Geometry: final body of the model. Coordinates: model frame, mm. Face numbers are marked on the shaded views. Round coordinates to 2 decimals unless told otherwise and drop trailing zeros. Loops run counter-clockwise (first coordinate to the right, second up) from the corner with the lowest first, then second, coordinate; pieces in that order, holes last. Notation, with made-up numbers: M -36,9 L 18,9 A13 ccw 18,17 Z; hole C 61,-14.75 d1. An arc over 180 degrees is marked long. Answer as a JSON object with one key per item and string values.
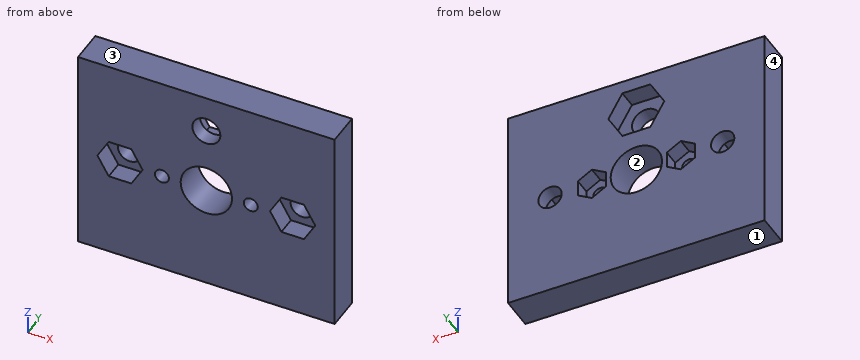
```python
from build123d import *

# Parameters (mm, degrees)
SKETCH1_W               = 55
SKETCH1_H               = 45
BOSS_EXTRUDE1_DEPTH     = 7.2
CUT_EXTRUDE1_DEPTH      = 37.253827384
CUT_EXTRUDE1_DEPTH_BACK = 37.253827384
SKETCH2_R               = 5.5
SKETCH2_R_2             = 2.5
SKETCH2_R_3             = 1.5
CUT_EXTRUDE2_DEPTH      = 3.5
CUT_EXTRUDE3_DEPTH      = 4
CUT_EXTRUDE4_DEPTH      = 37.253827384
CUT_EXTRUDE4_DEPTH_BACK = 37.253827384
SKETCH7_R               = 3
CUT_EXTRUDE5_DEPTH      = 4


with BuildPart() as part:
    # Sketch1 → Boss-Extrude1 (new body)
    with BuildSketch(Plane(origin=(0, 0, 0), x_dir=(1, 0, 0), z_dir=(0, 1, 0))):
        Rectangle(SKETCH1_W, SKETCH1_H)
    extrude(amount=BOSS_EXTRUDE1_DEPTH)

    # Sketch2 → Cut-Extrude1 (cut, two sides: drawn at the far end of the back side and taken through both)
    with BuildSketch(Plane(origin=(0, 7.2, 0), x_dir=(1, 0, 0), z_dir=(0, 1, 0)).offset(-CUT_EXTRUDE1_DEPTH_BACK)):
        with Locations(Location((0, 0, 0), (0, 0, 270))):
            Circle(SKETCH2_R)
        with Locations(Location((-18.5, 0, 0), (0, 0, 270))):
            Circle(SKETCH2_R_2)
        with Locations(Location((18.5, 0, 0), (0, 0, 270))):
            Circle(SKETCH2_R_2)
        with Locations(Location((-9.525, 0, 0), (0, 0, 270))):
            Circle(SKETCH2_R_3)
        with Locations(Location((9.525, 0, 0), (0, 0, 270))):
            Circle(SKETCH2_R_3)
    extrude(amount=CUT_EXTRUDE1_DEPTH + CUT_EXTRUDE1_DEPTH_BACK, mode=Mode.SUBTRACT)

    # Sketch3 → Cut-Extrude2 (cut)
    with BuildSketch(Plane(origin=(0, 7.2, 0), x_dir=(1, 0, 0), z_dir=(0, 1, 0))):
        Polygon((-9.525, 3.464101615), (-12.525, 1.732050808), (-12.525, -1.732050808), (-9.525, -3.464101615), (-6.525, -1.732050808), (-6.525, 1.732050808), align=None)
        Polygon((9.525, 3.464101615), (6.525, 1.732050808), (6.525, -1.732050808), (9.525, -3.464101615), (12.525, -1.732050808), (12.525, 1.732050808), align=None)
    extrude(amount=-CUT_EXTRUDE2_DEPTH, mode=Mode.SUBTRACT)

    # Sketch5 → Cut-Extrude3 (cut)
    with BuildSketch(Plane.XZ):
        Polygon((23.349742261, 0), (20.924871131, 4.2), (16.075128869, 4.2), (13.650257739, 0), (16.075128869, -4.2), (20.924871131, -4.2), align=None)
        Polygon((-13.650257739, 0), (-16.075128869, 4.2), (-20.924871131, 4.2), (-23.349742261, 0), (-20.924871131, -4.2), (-16.075128869, -4.2), align=None)
    extrude(amount=-CUT_EXTRUDE3_DEPTH, mode=Mode.SUBTRACT)

    # Sketch7 → Cut-Extrude4 (cut, two sides: drawn at the far end of the back side and taken through both)
    with BuildSketch(Plane(origin=(0, 7.2, 0), x_dir=(1, 0, 0), z_dir=(0, 1, 0)).offset(-CUT_EXTRUDE4_DEPTH_BACK)):
        with Locations(Location((0, -14.5, 0), (0, 0, 270))):
            Circle(SKETCH7_R)
    extrude(amount=CUT_EXTRUDE4_DEPTH + CUT_EXTRUDE4_DEPTH_BACK, mode=Mode.SUBTRACT)

    # Sketch8 → Cut-Extrude5 (cut)
    with BuildSketch(Plane(origin=(0, 7.2, 0), x_dir=(1, 0, 0), z_dir=(0, 1, 0))):
        Polygon((6.0044428, -14.5), (3.0022214, -9.3), (-3.0022214, -9.3), (-6.0044428, -14.5), (-3.0022214, -19.7), (3.0022214, -19.7), align=None)
    extrude(amount=-CUT_EXTRUDE5_DEPTH, mode=Mode.SUBTRACT)


solid = part.part
```
1) Line query: probe 1 along X at (y, z) = (4.75, 0) (3 decimals); probe 2 along X at (y, z) = (2.3, 0) (3 decimals); probe 3 along Z at (x, y) = (-3.5, 4.5). Output: solid intervals per line, ascending.
Geometry results:
{"probe 1": "-27.5 to -21, -16 to -12.525, -6.525 to -5.5, 5.5 to 6.525, 12.525 to 16, 21 to 27.5", "probe 2": "-27.5 to -23.35, -13.65 to -11.025, -8.025 to -5.5, 5.5 to 8.025, 11.025 to 13.65, 23.35 to 27.5", "probe 3": "-22.5 to -4.24, 4.24 to 10.16, 18.84 to 22.5"}
2) Pull-direction query (Z, two-part tool) for the marked faces 1, 2, 3 and 4; classes: +Z half, -Z half, draft (parallel to the pull), parting line (faces both ways), or undercut.
Geometry results:
{"face 1": "-Z half", "face 2": "undercut", "face 3": "+Z half", "face 4": "draft"}
3) Cut plane C-C on y = 1.75. Return the cut outline in (x, z) (3 decimals), and give its area (3 significant figures).
Geometry results:
{"outline": "M -27.5,-22.5 L 27.5,-22.5 L 27.5,22.5 L -27.5,22.5 Z; hole M -23.35,0 L -20.925,-4.2 L -16.075,-4.2 L -13.65,0 L -16.075,4.2 L -20.925,4.2 Z; hole C -9.525,0 d3; hole C 0,0 d11; hole C 0,14.5 d6; hole C 9.525,0 d3; hole M 13.65,0 L 16.075,-4.2 L 20.925,-4.2 L 23.35,0 L 20.925,4.2 L 16.075,4.2 Z", "area": "2,220 mm2"}
4) First-contact query: pin 1 (3 mm diameter, centred on x = 8.5, z = 1, fed in from +Y); pin 2 (8 mm diameter, centred on x = 1, z = 0.5, fed in from -Y); pin 3 (9 mm diameter, centred on x = -17, z = 2, fed in from -Y). Flat tips, straight axial feed; report the tip coordinate or a pass-through.
Geometry results:
{"pin 1": "y = 3.7", "pin 2": "through", "pin 3": "y = 0"}
5) Cut plane B-B on x = 18.5. Return the cut outline in (y, z), and give its area (3 significant figures).
Geometry results:
{"outline": "M 0,-22.5 L 7.2,-22.5 L 7.2,-2.5 L 4,-2.5 L 4,-4.2 L 0,-4.2 Z; M 0,4.2 L 4,4.2 L 4,2.5 L 7.2,2.5 L 7.2,22.5 L 0,22.5 Z", "area": "274 mm2"}
6) Cut plane A-A on x = 0. Return the cut outline in (y, z), and give its area (3 significant figures).
Geometry results:
{"outline": "M 0,-22.5 L 7.2,-22.5 L 7.2,-5.5 L 0,-5.5 Z; M 0,5.5 L 7.2,5.5 L 7.2,9.3 L 3.2,9.3 L 3.2,11.5 L 0,11.5 Z; M 0,17.5 L 3.2,17.5 L 3.2,19.7 L 7.2,19.7 L 7.2,22.5 L 0,22.5 Z", "area": "184 mm2"}
7) Cut plane D-D on y = 6.5. Return the cut outline in (x, z) (3 decimals), and give its area (3 significant figures).
Geometry results:
{"outline": "M -27.5,-22.5 L 27.5,-22.5 L 27.5,22.5 L -27.5,22.5 Z; hole C -18.5,0 d5; hole M -12.525,-1.732 L -9.525,-3.464 L -6.525,-1.732 L -6.525,1.732 L -9.525,3.464 L -12.525,1.732 Z; hole M -6.004,14.5 L -3.002,9.3 L 3.002,9.3 L 6.004,14.5 L 3.002,19.7 L -3.002,19.7 Z; hole C 0,0 d11; hole M 6.525,-1.732 L 9.525,-3.464 L 12.525,-1.732 L 12.525,1.732 L 9.525,3.464 L 6.525,1.732 Z; hole C 18.5,0 d5", "area": "2,180 mm2"}
